The listing builds one solid part. Answer for the finished solid, in the listing's coordinates (mm). A direction names the side the tool comes from. Coordinates: 2 decimals unless noted, no trailing zeros. Order: outer loops, then holes, each group sorted by start corner. A loop starts at its lowest first (then second) coordinate and runs counter-clockwise, first axis right, second up.
```python
from build123d import *

# Parameters (mm, degrees)
SKETCH1_R           = 3
BOSS_EXTRUDE1_DEPTH = 8.5
CUT_EXTRUDE1_DEPTH  = 6
SKETCH3_W           = 40
SKETCH3_H           = 6
BOSS_EXTRUDE2_DEPTH = 12.5
SKETCH4_R           = 1.55
CUT_EXTRUDE2_DEPTH  = 25.336187047
SKETCH6_W           = 8.25
SKETCH6_H           = 12.5
BOSS_EXTRUDE3_DEPTH = 9
SKETCH7_W           = 8.25
SKETCH7_H           = 5
CUT_EXTRUDE3_DEPTH  = 11.5


with BuildPart() as part:
    # Sketch1 → Boss-Extrude1 (new body)
    with BuildSketch(Plane(origin=(0, 0, 0), x_dir=(1, 0, 0), z_dir=(0, 1, 0))):
        with Locations(Location((0, 0, 0), (0, 0, 270))):
            Circle(SKETCH1_R)
    extrude(amount=BOSS_EXTRUDE1_DEPTH)

    # Sketch2 → Cut-Extrude1 (cut)
    with BuildSketch(Plane(origin=(0, 8.5, 0), x_dir=(1, 0, 0), z_dir=(0, 1, 0))):
        with BuildLine():
            Line((-1.101332519, -1.01836471), (1.134429265, -0.981361423))
            ThreePointArc((1.134429265, -0.981361423), (-0.02482256, 1.499794599), (-1.101332519, -1.01836471))
        make_face()
    extrude(amount=-CUT_EXTRUDE1_DEPTH, mode=Mode.SUBTRACT)

    # Sketch3 → Boss-Extrude2 (add)
    with BuildSketch(Plane.XZ):
        Rectangle(SKETCH3_W, SKETCH3_H)
    extrude(amount=BOSS_EXTRUDE2_DEPTH)

    # Sketch4 → Cut-Extrude2 (cut, through all)
    with BuildSketch(Plane(origin=(0, 0, -3), x_dir=(-1, 0, 0), z_dir=(0, 0, -1))):
        with Locations((15.5, -7.5)):
            Circle(SKETCH4_R)
    extrude(amount=-CUT_EXTRUDE2_DEPTH, mode=Mode.SUBTRACT)

    # Sketch6 → Boss-Extrude3 (add)
    with BuildSketch(Plane(origin=(0, 0, -3), x_dir=(-1, 0, 0), z_dir=(0, 0, -1))):
        with Locations((-15.875, -6.25)):
            Rectangle(SKETCH6_W, SKETCH6_H)
    extrude(amount=BOSS_EXTRUDE3_DEPTH)

    # Sketch7 → Cut-Extrude3 (cut)
    with BuildSketch(Plane.XZ.offset(12.5)):
        with Locations((15.875, -5.5)):
            Rectangle(SKETCH7_W, SKETCH7_H)
    extrude(amount=-CUT_EXTRUDE3_DEPTH, mode=Mode.SUBTRACT)


solid = part.part
```
(1) Find section B-B (y = -7.5). Write down the section's boundary in (x, z).
(2) Consider line 1 (Y direction, x = -15.5, z = -0.7); line 2 (X direction, y = 6.6, z = 0); line 3 (Z direction, x = 9.5, y = -0.5). Determine where each line is inside the solid, lowest interval first.
(3) Each of these flat-tipped pins is pushed along its axis until it touches: pin 1 Ø1.5 at (x, y) = (3.5, -2.5) entering from -Z; pin 2 Ø1.5 at (y, z) = (2.5, -1) entering from -X; pin 3 Ø2.5 at (x, z) = (16, -5) entering from -Y. Where does it stop, or does it pass through?
(4) Find section C-C (z = 0). Write down the section's boundary in (x, y).
(5) Find section D-D (y = -4.25). Write down the section's boundary in (x, z), and give its area (3 significant figures).
(6) For faces 1 (the face through (-20, -6, 0)), 2 (the face through (11.75, -6, -9)), 3 (the face through (16, -7, -8)), 4 (the face through (0, 2.5, 0)), determine the directions among +Z, -Z, +X, -X, +Y, -Y from which every point of the face is accessible in a straight line to the end or side of a thin tool.
(7) The mould has two halves that part along Y. Classify faces 5 (the face through (20, -6.3, -2.7)), 6 (the face through (-12, 0, 0)), 7 (the face through (-14.27, -8.44, -0.04)): released by +Y, released by -Y, zero draft, split by the parting line, or undercut.
(8) Find section A-A (x = -15.5). Write down the section's boundary in (y, z), and give its area (3 significant figures).
Findings below:
1. outline: (-20, -3) - (-17.05, -3) - (-17.05, 3) - (-20, 3) - close; (-13.95, -3) - (20, -3) - (20, 3) - (-13.95, 3) - close; (11.75, -12) - (20, -12) - (20, -8) - (11.75, -8) - close
2. line 1: y = -12.5 to -9.05, -5.95 to 0
2. line 2: x = -3 to -1.5, 1.5 to 3
2. line 3: z = -3 to 3
3. pin 1: stops at z = -3
3. pin 2: stops at x = -2.99
3. pin 3: stops at y = -1
4. outline: (-20, -12.5) - (20, -12.5) - (20, 0) - (3, 0) - (3, 8.5) - (1.5, 8.5) - (1.5, 2.5) - (-1.5, 2.5) - (-1.5, 8.5) - (-3, 8.5) - (-3, 0) - (-20, 0) - close; hole circle Ø3.1 at (-15.5, -7.5)
5. outline: (-20, -3) - (20, -3) - (20, 3) - (-20, 3) - close; (11.75, -12) - (20, -12) - (20, -8) - (11.75, -8) - close
5. area: 273 mm2
6. face 1: +Z, -Z, -X, +Y, -Y
6. face 2: -Z, -X, +Y, -Y
6. face 3: +X, -X, -Y
6. face 4: +Y
7. face 5: zero draft
7. face 6: released by +Y
7. face 7: undercut
8. outline: (-12.5, -3) - (-9.05, -3) - (-9.05, 3) - (-12.5, 3) - close; (-5.95, -3) - (0, -3) - (0, 3) - (-5.95, 3) - close
8. area: 56.4 mm2
